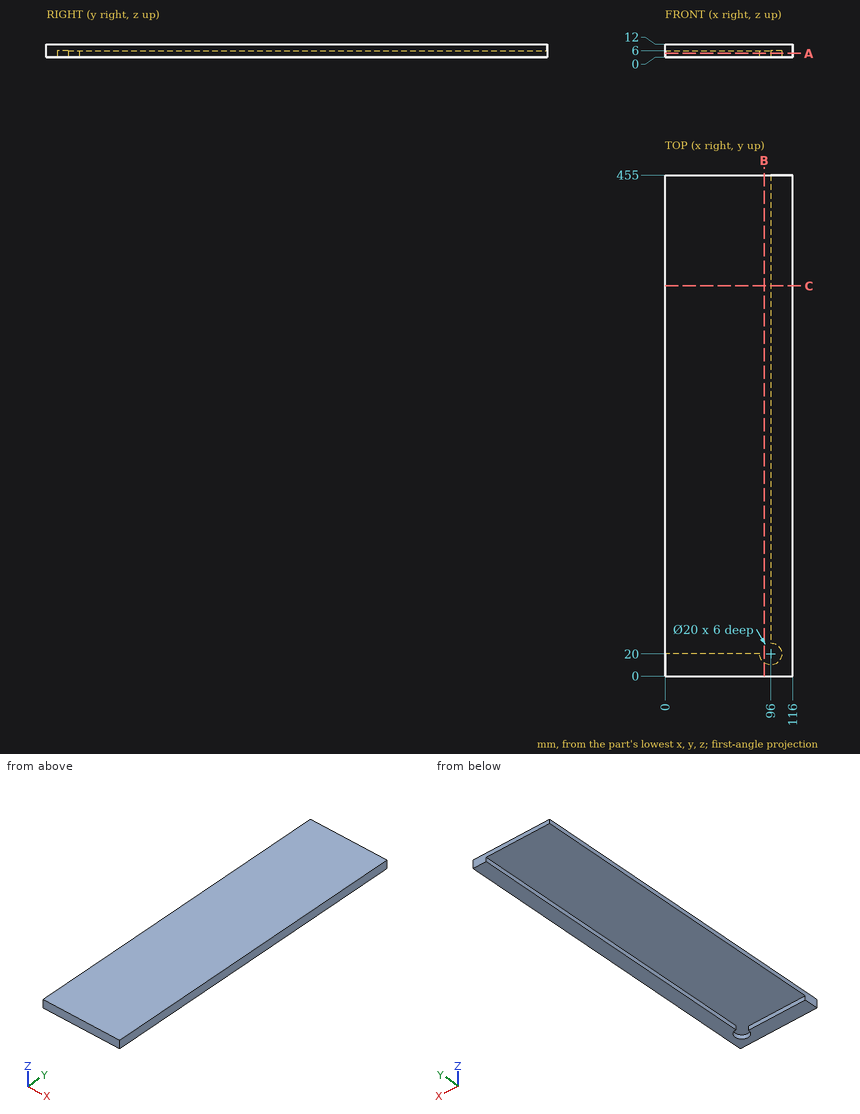
Job drawing, mm, ordinate dimensions from the low corner. One solid piece. Coordinates: 2 decimals unless noted, no trailing zeros. Write each loop counter-clockwise with the first axis right and the second up, starting at its lowest first coordinate (ties: lowest second). Pieces come first, ordered by that corner, then holes.
Item 1: Probe line 1 (Z direction, x = 62.5, y = 43.5); line 2 (X direction, y = 111.5, z = 3.5); line 3 (Y direction, x = 102.5, z = 1.25). List the from-to ranges inside material, lowest first.
Item 2: Slice it at B-B (x = 90). Write the cut outline in (y, z), and give its area (3 significant figures).
Item 3: Slice it at A-A (z = 3.5). Write the cut outline in (x, y), and give its area (3 significant figures).
Item 4: Pin check, flat tips, straight feed: pin 1 (1.5 mm diameter, centred on x = 48, z = 7.5, fed in from -Y); pin 2 (1.8 mm diameter, centred on y = 231.5, z = 3, fed in from -X); pin 3 (5 mm diameter, centred on x = 28, z = 2, fed in from +Y); pin 4 (10 mm diameter, centred on x = 55.5, y = 328, fed in from -Z). Stop position of each tip, or through.
Item 5: Slice it at C-C (y = 354.5). Write the cut outline in (x, z).
Results found:
1. line 1: z = 6 to 12
1. line 2: x = 96 to 116
1. line 3: y = 0 to 12.4, 27.6 to 455
2. outline: (0, 0) - (12, 0) - (12, 6) - (455, 6) - (455, 12) - (0, 12) - close
2. area: 2,800 mm2
3. outline: (0, 0) - (116, 0) - (116, 455) - (96, 455) - (96, 30) arc R10 cw (long way) to (86, 20) - (0, 20) - close
3. area: 10,800 mm2
4. pin 1: stops at y = 0
4. pin 2: stops at x = 96
4. pin 3: stops at y = 20
4. pin 4: stops at z = 6
5. outline: (0, 6) - (96, 6) - (96, 0) - (116, 0) - (116, 12) - (0, 12) - close
